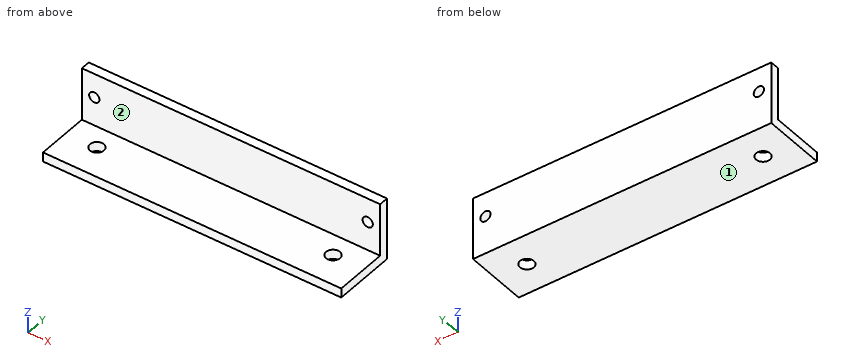
from build123d import *

# Parameters (mm, degrees)
SKETCH_1_W           = 96
SKETCH_1_H           = 20
EXTRUDE_1_DEPTH      = 3
SKETCH_2_W           = 96
SKETCH_2_H           = 3
EXTRUDE_2_DEPTH      = 17
HOLE_WIZARD_M4_1_D   = 4.5
HOLE_WIZARD_M4_1_2_D = 3.3


with BuildPart() as part:
    # 스케치1 → 보스-돌출1 (new body)
    with BuildSketch(Plane.XY):
        Rectangle(SKETCH_1_W, SKETCH_1_H)
    extrude(amount=EXTRUDE_1_DEPTH)

    # 스케치2 → 보스-돌출2 (add)
    with BuildSketch(Plane.XY.offset(3)):
        with Locations((0, 8.5)):
            Rectangle(SKETCH_2_W, SKETCH_2_H)
    extrude(amount=EXTRUDE_2_DEPTH)

    # Hole Wizard M4 _ _1 (through all)
    with Locations(Plane.XY.offset(3)):
        with Locations((-38, 0), (38, 0)):
            Hole(HOLE_WIZARD_M4_1_D / 2)

    # Hole Wizard M4 _ _1 2 (through all)
    with Locations(Plane(origin=(0, 10, 0), x_dir=(1, 0, 0), z_dir=(0, 1, 0))):
        with Locations((-44, -12.25), (44, -12.25)):
            Hole(HOLE_WIZARD_M4_1_2_D / 2)


solid = part.part
Work out the finished part from the listing and answer in its coordinate system (mm). Face numbers are marked on the shaded views. A direction names the side the tool comes from. Give positions to 0.01 mm unless a question says otherwise; leave off trailing zeros. Write each loop counter-clockwise with the first axis right and the second up, starting at its lowest first coordinate (ties: lowest second). Pieces come first, ordered by that corner, then holes. Notation, with made-up numbers: (-14.5, 10.25) - (37.5, 10.25) arc R16 cw to (37.5, 37.25) - close; hole circle Ø6 at (-31.5, -38). An arc over 180 degrees is marked (long way). One line per item, written item: value. Start each with the question number.
1. For the marked faces 1 and 2, determine the directions among +Z, -Z, +X, -X, +Y, -Y from which every point of the face is accessible in a straight line to the end or side of a thin tool.
2. Given pin 1 (3.5 mm diameter, centred on x = 38, y = 0, fed in from -Z); pin 2 (5 mm diameter, centred on x = 12.5, z = 10, fed in from -Y); pin 3 (8.5 mm diameter, centred on x = -14.5, y = 1.5, fed in from +Z), each flat-ended and moving along its own axis, determine where each tip first touches the part or whether it passes through.
3. Find section A-A (x = -44). Write down the section's boundary in (y, z).
4. Consider probe 1 along X at (y, z) = (9.3, 12.25); probe 2 along Z at (x, y) = (-44, 7.8); probe 3 along Y at (x, z) = (-38, 0.75). Determine where each line is inside the solid, lowest interval first.
5. Find section D-D (z = 1.5). Write down the section's boundary in (x, y).
6. Find section C-C (z = 12.25). Write down the section's boundary in (x, y).
7. Find section B-B (y = 0). Write down the section's boundary in (x, z).
Geometry results:
1. face 1: -Z, +X, -X, +Y, -Y
1. face 2: +Z, +X, -X, -Y
2. pin 1: through
2. pin 2: y = 7
2. pin 3: z = 3
3. outline: (-10, 0) - (10, 0) - (10, 10.6) - (7, 10.6) - (7, 3) - (-10, 3) - close; (7, 13.9) - (10, 13.9) - (10, 20) - (7, 20) - close
4. probe 1: -48 to -45.65, -42.35 to 42.35, 45.65 to 48
4. probe 2: 0 to 10.6, 13.9 to 20
4. probe 3: -10 to -2.25, 2.25 to 10
5. outline: (-48, -10) - (48, -10) - (48, 10) - (-48, 10) - close; hole circle Ø4.5 at (-38, 0); hole circle Ø4.5 at (38, 0)
6. outline: (-48, 7) - (-45.65, 7) - (-45.65, 10) - (-48, 10) - close; (-42.35, 7) - (42.35, 7) - (42.35, 10) - (-42.35, 10) - close; (45.65, 7) - (48, 7) - (48, 10) - (45.65, 10) - close
7. outline: (-48, 0) - (-40.25, 0) - (-40.25, 3) - (-48, 3) - close; (-35.75, 0) - (35.75, 0) - (35.75, 3) - (-35.75, 3) - close; (40.25, 0) - (48, 0) - (48, 3) - (40.25, 3) - close
